Can you work these out from the model? Positions are in its coordinate system, mm. Face numbers are marked on the shaded views. A direction names the side the tool comes from. Give positions to 0.01 mm unless a question says otherwise; leave off trailing zeros. Order: outer loops, then holes, each group sorted by start corner. A loop starts at its lowest first (then second) coordinate and runs counter-clockwise, first axis right, second up. Notation, with made-up numbers: (11.25, 18.5) - (68.25, 18.5) arc R30 ccw to (68.25, 49.5) - close; hole circle Ø9 at (56, 72). An arc over 180 degrees is marked (long way). Answer as CSV lines item,"result".
Autodesk Inventor part; units mm, degrees
ref_plane "作業平面1" through (10, 0, 0) normal (1, 0, 0) x (0, 1, 0)
ref_plane "XZ Plane" through (0, 0, 0) normal (0, 1, 0) x (-1, 0, 0)
ref_plane "XY Plane" through (0, 0, 0) normal (0, 0, 1) x (1, 0, 0)
sketch "スケッチ1" plane through (0, 0, 0) normal (0, 0, 1) x (1, 0, 0)
  line L0 (2.8284, 0) -> (0, -2.8284)
  line L1 (0, -2.8284) -> (-2.8284, 0)
  line L2 (-2.8284, 0) -> (0, 2.8284)
  line L3 (0, 2.8284) -> (2.8284, 0)
  line L4 (-12.1149, 7.5) -> (-10, -7.5)
  line L5 (10, -7.5) -> (-10, -7.5)
  line L6 (10, -7.5) -> (12.1149, 7.5)
  line L7 (12.1149, 7.5) -> (-12.1149, 7.5)
  point P0 (0, 0)
  point P1 (0, 7.5)
  point P2 (11.0574, 0)
  dimension "d10" = 24.2298
  dimension "d11" = 20
  dimension "d12" = 15
  dimension "d13" = 4
extrude "押し出し1" add sketch "スケッチ1" against normal blind 2
ref_plane "作業平面1" through (10, 0, 0) normal (1, 0, 0) x (0, 1, 0)
sketch "スケッチ3" plane through (10, 0, 0) normal (1, 0, 0) x (0, 1, 0)
  line L0 (7.5, 0) -> (-7.5, 0)
  line L1 (7.5, 0) -> (7.5, -2)
  line L2 (-7.5, -2) -> (7.5, -2)
  line L3 (-7.5, 0) -> (-7.5, -2)
  line L4 (7.5, -2) -> (2.254, -4.912)
  line L5 (1.6578, -4.1213) -> (3.7791, -2)
  arc A0 (1.6578, -4.1213) -> (2.254, -4.912) centre (2.0114, -4.4749) ccw
  point P0 (0, 0)
  dimension "d17" = 0.5
  dimension "d18" = 45
  dimension "d19" = 6
  dimension "d25" = 3
extrude "押し出し3" add sketch "スケッチ3" against normal blind 2 contours L4 A0 L5 L2
fillet "フィレット1" radius 1 2 edges at (10, 5.6396, -2) (8, 5.6396, -2)
fillet "フィレット2" radius 0.5 2 edges at (7.5, 3.7791, -2) (10.5, 3.7791, -2)
mirror "ミラー2" about plane through (0, 0, 0) normal (1, 0, 0) of "押し出し3", "フィレット1", "フィレット2"
properties part number "om_BackHolder_V4"
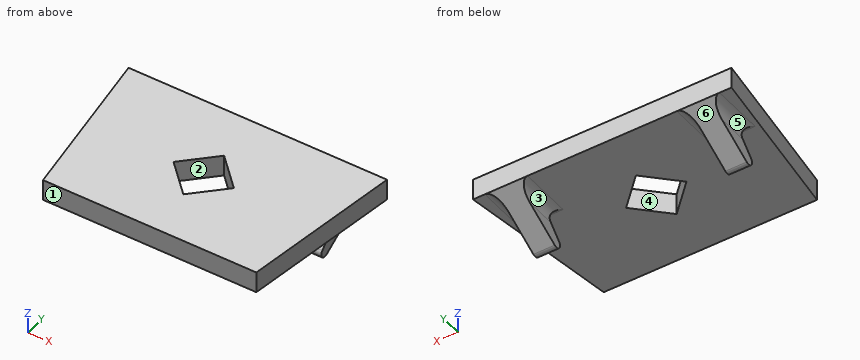
1) I want a section at B-B on x = 0.25. Write out the boundary of the cut face in (y, z), plus the area to 3 significant figures.
Answer block:
outline,"(-7.5, -2) - (-2.58, -2) - (-2.58, 0) - (-7.5, 0) - close; (2.58, -2) - (7.5, -2) - (7.5, 0) - (2.58, 0) - close"
area,"19.7 mm2"
2) I want a section at C-C on z = -0.9. Write out the boundary of the cut face in (x, y).
Answer block:
outline,"(-12.11, 7.5) - (-10, -7.5) - (10, -7.5) - (12.11, 7.5) - close; hole (-2.83, 0) - (0, -2.83) - (2.83, 0) - (0, 2.83) - close"
3) I'm going to push flat-ended pins straight in: P1, Ø1, axis at y = -3.5, z = -4, coming from the -X side; P2, Ø1, axis at y = 3.5, z = -4, coming from the -X side; P3, Ø1, axis at x = 7, y = -4.5, coming from the -Z side; P4, Ø0.6, axis at y = 3, z = -4, coming from the +X side. Where does each tip first touch, or does it pass through?
Answer block:
P1,"through"
P2,"x = -10"
P3,"z = -2"
P4,"x = 10"
4) If we mould it in two halves opening along Y, with no side actions, what happens to the marked faces 4, 5 and 6? For each: +Y half, -Y half, draft (parallel to the pull), parting line (faces both ways), or undercut.
Answer block:
face 4,"undercut"
face 5,"draft"
face 6,"+Y half"
5) I want a section at A-A on y = -1.5. Write out the boundary of the cut face in (x, z), plus the area to 3 significant figures.
Answer block:
outline,"(-10.85, -2) - (-1.33, -2) - (-1.33, 0) - (-10.85, 0) - close; (1.33, -2) - (10.85, -2) - (10.85, 0) - (1.33, 0) - close"
area,"38.1 mm2"
6) I want a section at D-D on y = 6. Write out the boundary of the cut face in (x, z).
Answer block:
outline,"(-11.9, -2) - (-11, -2) arc R1 cw to (-10.01, -2.83) - (-7.99, -2.83) arc R1 cw to (-7, -2) - (7, -2) arc R1 cw to (7.99, -2.83) - (10.01, -2.83) arc R1 cw to (11, -2) - (11.9, -2) - (11.9, 0) - (-11.9, 0) - close"
7) I need wall thicknesses on line 1 along X through (y, z) = (2.25, -4.1); line 2 along Z through (x, y) = (9.25, -3.25); line 3 along X through (y, z) = (-2.5, -1.95). Which ranges of each line are inside material? Lowest first, please. Write a range as [from, to].
Answer block:
line 1,"[-10, -8], [8, 10]"
line 2,"[-2, 0]"
line 3,"[-10.7, -0.33], [0.33, 10.7]"
8) Which directions (+Z, -Z, +X, -X, +Y, -Y) give clear straight access to the entire face, cutting with the end or side of a thin tool? Please do the marked faces 1, 2 and 3.
Answer block:
face 1,"+Z, -Z, +X, -X, -Y"
face 2,"+Z, -Z"
face 3,"-Z, +Y, -Y"
